from build123d import *

# Parameters (mm, degrees)
BOSS_EXTRUDE1_DEPTH     = 17
SKETCH2_R               = 2.5
BOSS_EXTRUDE2_DEPTH     = 1
CUT_EXTRUDE1_DEPTH      = 3
CUT_EXTRUDE5_DEPTH      = 2
CUT_EXTRUDE5_DEPTH_BACK = 3
SKETCH5_W               = 1.356176493
SKETCH5_H               = 3
CUT_EXTRUDE6_DEPTH      = 3
CUT_EXTRUDE11_DEPTH     = 20
CUT_EXTRUDE12_DEPTH     = 1
SKETCH12_W              = 28
SKETCH12_H              = 17
BOSS_EXTRUDE3_DEPTH     = 2
SKETCH13_W              = 28
SKETCH13_H              = 17
BOSS_EXTRUDE4_DEPTH     = 2
SKETCH14_W              = 1.356176493
SKETCH14_H              = 14
BOSS_EXTRUDE5_DEPTH     = 1
SKETCH15_W              = 1.356176493
SKETCH15_H              = 14
BOSS_EXTRUDE6_DEPTH     = 1
BOSS_EXTRUDE7_DEPTH     = 1
BOSS_EXTRUDE8_DEPTH     = 1
SKETCH18_W              = 1.356176493
SKETCH18_H              = 14
BOSS_EXTRUDE9_DEPTH     = 2
SKETCH19_W              = 1.356176493
SKETCH19_H              = 14
BOSS_EXTRUDE10_DEPTH    = 2


with BuildPart() as part:
    # Sketch1 → Boss-Extrude1 (new body)
    with BuildSketch(Plane(origin=(0, 0, 0), x_dir=(1, 0, 0), z_dir=(0, 1, 0))):
        Polygon((53.231444905, 93.562909441), (55.368661466, 80.762909441), (59.368661466, 80.762909441), (59.368661466, 66.562909441), (55.368661466, 66.562909441), (53.231444905, 53.762909441), (25.231444905, 53.762909441), (25.231444905, 58.012909441), (42.701133317, 58.012909441), (42.701133317, 66.512909441), (41.344956824, 66.512909441), (41.344956824, 70.012909441), (12.018661466, 71.012909441), (12.018661466, 76.312909441), (41.344956824, 77.312909441), (41.344956824, 80.812909441), (42.701133317, 80.812909441), (42.701133317, 89.312909441), (25.231444905, 89.312909441), (25.231444905, 93.562909441), align=None)
    extrude(amount=BOSS_EXTRUDE1_DEPTH)

    # Sketch2 → Boss-Extrude2 (add)
    with BuildSketch(Plane.XZ):
        with Locations((42.701133317, -73.662909441)):
            Circle(SKETCH2_R)
    extrude(amount=BOSS_EXTRUDE2_DEPTH)

    # Sketch3 → Cut-Extrude1 (cut)
    with BuildSketch(Plane(origin=(0, 0, 0), x_dir=(-1, 0, 0), z_dir=(0, -1, 0))):
        with BuildLine():
            Line((-42.701133317, 80.812909441), (-55.368661466, 80.762909441))
            Line((-55.368661466, 80.762909441), (-59.368661466, 80.762909441))
            Line((-59.368661466, 80.762909441), (-59.368661466, 66.562909441))
            Line((-59.368661466, 66.562909441), (-41.344956824, 66.512909441))
            Line((-41.344956824, 66.512909441), (-41.344956824, 70.012909441))
            Line((-41.344956824, 70.012909441), (-41.344956824, 71.562722468))
            ThreePointArc((-41.344956824, 71.562722468), (-45.201133317, 73.662909441), (-41.344956824, 75.763096414))
            Line((-41.344956824, 75.763096414), (-41.344956824, 77.312909441))
            Line((-41.344956824, 77.312909441), (-41.344956824, 80.812909441))
            Line((-41.344956824, 80.812909441), (-42.701133317, 80.812909441))
        make_face()
    extrude(amount=-CUT_EXTRUDE1_DEPTH, mode=Mode.SUBTRACT)

    # Sketch4 → Cut-Extrude5 (cut, two sides)
    with BuildSketch(Plane.XZ) as cut_extrude5_sk:
        with BuildLine():
            Line((12.018661466, -76.312909441), (41.344956824, -77.312909441))
            Line((41.344956824, -77.312909441), (41.344956824, -77.220900459))
            Line((41.344956824, -77.220900459), (41.344956824, -75.763096414))
            ThreePointArc((41.344956824, -75.763096414), (40.201133317, -73.662909441), (41.344956824, -71.562722468))
            Line((41.344956824, -71.562722468), (41.344956824, -70.012909441))
            Line((41.344956824, -70.012909441), (12.018661466, -71.012909441))
            Line((12.018661466, -71.012909441), (12.018661466, -76.312909441))
        make_face()
    extrude(amount=CUT_EXTRUDE5_DEPTH, mode=Mode.SUBTRACT)
    extrude(cut_extrude5_sk.sketch, amount=-CUT_EXTRUDE5_DEPTH_BACK, mode=Mode.SUBTRACT)

    # Sketch5 → Cut-Extrude6 (cut)
    with BuildSketch(Plane.XY.offset(-66.512909441)):
        with Locations((42.023045071, 1.5)):
            Rectangle(SKETCH5_W, SKETCH5_H)
    extrude(amount=-CUT_EXTRUDE6_DEPTH, mode=Mode.SUBTRACT)

    # Sketch7 → Cut-Extrude11 (cut)
    with BuildSketch(Plane.ZY.offset(-42.701133317)):
        Polygon((-66.516671643, 0), (-67.290586566, 0), (-67.290586566, 3), (-66.512909441, 3), (-58.012909441, 0), align=None)
        Polygon((-89.312909441, 0), (-80.812909441, 0), (-79.713237651, 0), (-79.713237651, 3), (-80.812909441, 3), align=None)
    extrude(amount=-CUT_EXTRUDE11_DEPTH, mode=Mode.SUBTRACT)

    # Sketch11 → Cut-Extrude12 (cut)
    with BuildSketch(Plane.XZ.offset(-3)):
        with BuildLine():
            Line((41.344956824, -77.312909441), (41.344956824, -75.763096414))
            ThreePointArc((41.344956824, -75.763096414), (40.201133317, -73.662909441), (41.344956824, -71.562722468))
            Line((41.344956824, -71.562722468), (41.344956824, -70.012909441))
            Line((41.344956824, -70.012909441), (12.018661466, -71.012909441))
            Line((12.018661466, -71.012909441), (12.018661466, -76.312909441))
            Line((12.018661466, -76.312909441), (41.344956824, -77.312909441))
        make_face()
    extrude(amount=-CUT_EXTRUDE12_DEPTH, mode=Mode.SUBTRACT)

    # Sketch12 → Boss-Extrude3 (add)
    with BuildSketch(Plane(origin=(0, 0, -93.562909441), x_dir=(-1, 0, 0), z_dir=(0, 0, -1))):
        with Locations((-39.231444905, 8.5)):
            Rectangle(SKETCH12_W, SKETCH12_H)
    extrude(amount=BOSS_EXTRUDE3_DEPTH)

    # Sketch13 → Boss-Extrude4 (add)
    with BuildSketch(Plane.XY.offset(-53.762909441)):
        with Locations((39.231444905, 8.5)):
            Rectangle(SKETCH13_W, SKETCH13_H)
    extrude(amount=BOSS_EXTRUDE4_DEPTH)

    # Sketch14 → Boss-Extrude5 (add)
    with BuildSketch(Plane.XY.offset(-66.512909441)):
        with Locations((42.023045071, 10)):
            Rectangle(SKETCH14_W, SKETCH14_H)
    extrude(amount=BOSS_EXTRUDE5_DEPTH)

    # Sketch15 → Boss-Extrude6 (add)
    with BuildSketch(Plane(origin=(0, 0, -80.812909441), x_dir=(-1, 0, 0), z_dir=(0, 0, -1))):
        with Locations((-42.023045071, 10)):
            Rectangle(SKETCH15_W, SKETCH15_H)
    extrude(amount=BOSS_EXTRUDE6_DEPTH)

    # Sketch16 → Boss-Extrude7 (add)
    with BuildSketch(Plane.XY.offset(-66.562909441)):
        Polygon((59.368661466, 3), (55.368661466, 3), (53.667179365, 3), (53.667179365, 17), (55.368661466, 17), (59.368661466, 17), align=None)
    extrude(amount=BOSS_EXTRUDE7_DEPTH)

    # Sketch17 → Boss-Extrude8 (add)
    with BuildSketch(Plane(origin=(0, 0, -80.762909441), x_dir=(-1, 0, 0), z_dir=(0, 0, -1))):
        Polygon((-59.368661466, 3), (-55.368661466, 3), (-53.078047716, 3), (-53.078047716, 17), (-55.368661466, 17), (-59.368661466, 17), align=None)
    extrude(amount=BOSS_EXTRUDE8_DEPTH)

    # Sketch18 → Boss-Extrude9 (add)
    with BuildSketch(Plane.XY.offset(-65.512909441)):
        with Locations((42.023045071, 10)):
            Rectangle(SKETCH18_W, SKETCH18_H)
    extrude(amount=BOSS_EXTRUDE9_DEPTH)

    # Sketch19 → Boss-Extrude10 (add)
    with BuildSketch(Plane(origin=(0, 0, -81.812909441), x_dir=(-1, 0, 0), z_dir=(0, 0, -1))):
        with Locations((-42.023045071, 10)):
            Rectangle(SKETCH19_W, SKETCH19_H)
    extrude(amount=BOSS_EXTRUDE10_DEPTH)


solid = part.part
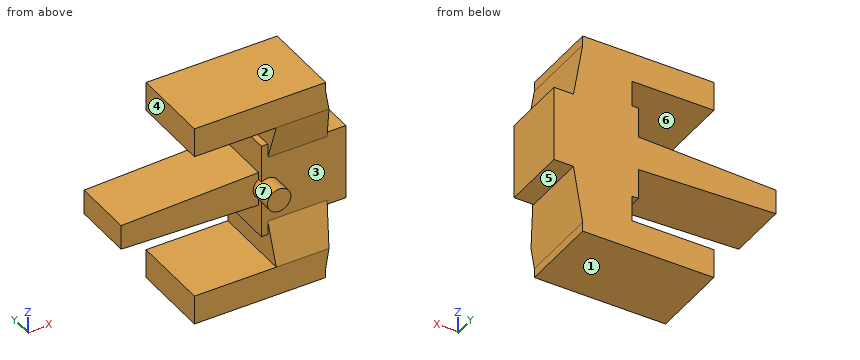
Can you work these out from the model? Positions are in its coordinate system, mm. Face numbers are marked on the shaded views. A direction names the side the tool comes from. Coordinates: 2 decimals unless noted, no trailing zeros. Loops run counter-clockwise (first coordinate to the right, second up) from the corner with the lowest first, then second, coordinate; pieces in that order, holes last. Notation, with made-up numbers: M 37.25,-30 L 44.25,-30 A11 cw 44.25,-17 Z; hole C 46,-19.5 d10. An arc over 180 degrees is marked long. Answer as CSV lines item,"result". Start each with the question number.
1. Suppose I cut it at A-A, the plane x = 34.5. List the corners of the cut face in (y, z) for me.
2. If I drill on probe 1 along Z at (x, y) = (42, 5.75); probe 2 along Z at (x, y) = (40.5, 10.5); probe 3 along Z at (x, y) = (40, 1.75), over which ranges is the centre line in solid material (lowest first)? Write a range as [from, to].
3. Suppose I cut it at C-C, the plane y = 15.25. List the corners of the cut face in (x, z) for me, plus the area to 3 significant figures.
4. Suppose I cut it at D-D, the plane z = -55. List the corners of the cut face in (x, y) for me, plus the area to 3 significant figures.
5. Thinking about a two-plate mould opening in Z: for the marked faces 1, 2 and 3, which applies, +Z half, -Z half, draft (parallel to the pull), parting line (faces both ways), or undercut?
6. For the marked faces 4, 5, 6 and 7, which set-ups out of +Z, -Z, +X, -X, +Y, -Y let a thin tool reach every point of the face, with its end or its side?
7. For pin 1 Ø3.5 at (x, y) = (57.5, 11.5) entering from -Z; pin 2 Ø1 at (y, z) = (4.5, -53) entering from +X; pin 3 Ø5 at (x, z) = (51, -76) entering from -Y, each with a flat end and sliding along its axis, tell me the tip position at first contact or that it passes through.
8. Suppose I cut it at B-B, the plane x = 49. List the corners of the cut face in (y, z) for me, plus the area to 3 significant figures.
Output:
1,outline,"M 0,-95.56 L 17,-95.56 L 17,-89.31 L 0,-89.31 Z; M 0,-58.01 L 17,-58.01 L 17,-51.76 L 0,-51.76 Z; M 4,-77.08 L 17,-77.08 L 17,-70.25 L 4,-70.25 Z"
2,probe 1,"z = [-95.56, -89.31], [-83.81, -63.51], [-58.01, -51.76]"
2,probe 2,"z = [-95.56, -89.31], [-77.28, -70.04], [-58.01, -51.76]"
2,probe 3,"z = [-95.56, -89.31], [-58.01, -51.76]"
3,outline,"M 12.02,-76.31 L 41.34,-77.31 L 41.34,-83.81 L 42.7,-83.81 L 42.7,-89.31 L 25.23,-89.31 L 25.23,-95.56 L 53.23,-95.56 L 53.23,-93.56 L 55.2,-81.76 L 59.37,-81.76 L 59.37,-65.56 L 55.2,-65.56 L 53.23,-53.76 L 53.23,-51.76 L 25.23,-51.76 L 25.23,-58.01 L 42.7,-58.01 L 42.7,-63.51 L 41.34,-63.51 L 41.34,-70.01 L 12.02,-71.01 Z"
3,area,"1,010 mm^2"
4,outline,"M 25.23,0 L 53.44,0 L 53.44,17 L 25.23,17 Z"
4,area,"480 mm^2"
5,face 1,"-Z half"
5,face 2,"+Z half"
5,face 3,"undercut"
6,face 4,"+Z, -X, +Y, -Y"
6,face 5,"-Z, +X, +Y, -Y"
6,face 6,"-X, +Y, -Y"
6,face 7,"-Y"
7,pin 1,"stops at z = -81.76"
7,pin 2,"stops at x = 53.23"
7,pin 3,"stops at y = 3"
8,outline,"M 0,-95.56 L 17,-95.56 L 17,-51.76 L 0,-51.76 L 0,-58.01 L 3,-66.51 L 3,-80.81 L 0,-89.31 Z"
8,area,"676 mm^2"
